Here's how the part is built. I have some questions about the finished solid (model axes, mm). A direction names the side the tool comes from. Coordinates: 2 decimals unless noted, no trailing zeros. Write each loop counter-clockwise with the first axis right and the second up, starting at its lowest first coordinate (ties: lowest second). Pieces come first, ordered by that corner, then holes.
Item 1: I want a section at A-A (x = -2). Please give me the cut outline in (y, z).
Item 2: I want a section at D-D (z = 19). Please give me the cut outline in (x, y).
Item 3: I'm going to push flat-ended pins straight in: P1, Ø5, axis at x = -6, z = -18.5, coming from the +Y side; P2, Ø6, axis at x = -18.5, z = 17, coming from the +Y side; P3, Ø11, axis at y = 12, z = 3, coming from the -X side; P4, Ø10, axis at x = -8.5, y = -3, coming from the -Z side. Where does each tip first touch, or does it pass through?
Item 4: If we mould it in two halves opening along Z, with no side actions, what happens to faces 4 (the face through (22.01, -2.96, -0.33)), 5 (the face through (0, 17, 6.5)), 6 (the face through (-0.28, 9.12, -13.9))? For each: pulls with the +Z half, pulls with the -Z half, needs draft (parallel to the pull), parting line crosses it, or undercut.
Item 5: For faces 1 (the face through (17.46, 7.03, 0.28)), 2 (the face through (-0.3, -2.96, -19.71)), 3 (the face through (11, 13, 0)), which set-ups out of +Z, -Z, +X, -X, +Y, -Y let a thin tool reach every point of the face, with its end or its side?
Item 6: Please list where these lines run through material, in increasing order: line 1 (Z direction, x = 8, y = -0.5); line 2 (Z direction, x = 19, y = -3.25); line 3 (X direction, y = 3, z = 15).
Item 7: I want a section at C-C (y = 5.75). Please give me the cut outline in (x, z), and give its area (3 significant figures).
Item 8: I want a section at B-B (z = -3.5). Please give me the cut outline in (x, y).
from build123d import *
from OCP.BRepFilletAPI import BRepFilletAPI_MakeChamfer

# Parameters (mm, degrees)
SKETCH1_W               = 40
SKETCH1_H               = 40
BOSS_EXTRUDE1_DEPTH     = 8.5
BOSS_EXTRUDE1_TAPER     = 40
SKETCH2_W               = 36
SKETCH2_H               = 36
CUT_EXTRUDE1_DEPTH      = 15
CUT_EXTRUDE1_DRAFT      = -40
SKETCH4_W               = 25.73530627
SKETCH4_H               = 25.73530627
BOSS_EXTRUDE3_DEPTH     = 10
SKETCH5_W               = 22
SKETCH5_H               = 13
CUT_EXTRUDE2_DEPTH      = 31.000000133
CHAMFER2_SIZE           = 12
CHAMFER2_SIZE_2         = 9.89892863
CUT_EXTRUDE3_DEPTH      = 35.154586706
CUT_EXTRUDE3_DEPTH_BACK = 35.154586706
CHAMFER3_SIZE           = 4.3
CHAMFER3_SIZE2          = 7.447818473
CUT_EXTRUDE4_DEPTH      = 35.154586706
CUT_EXTRUDE4_DEPTH_BACK = 35.154586706
SKETCH9_W               = 40.602605658
SKETCH9_H               = 40
BOSS_EXTRUDE4_DEPTH     = 6
BOSS_EXTRUDE4_DRAFT     = -30
SKETCH10_W              = 36.602605658
SKETCH10_H              = 36
CUT_EXTRUDE5_DEPTH      = 10
CUT_EXTRUDE5_DRAFT      = 30


with BuildPart() as part:
    # Sketch1 → Boss-Extrude1 (new body)
    with BuildSketch(Plane(origin=(0, 0, 0), x_dir=(1, 0, 0), z_dir=(0, 1, 0))):
        Rectangle(SKETCH1_W, SKETCH1_H)
    extrude(amount=BOSS_EXTRUDE1_DEPTH, taper=BOSS_EXTRUDE1_TAPER)


with BuildPart() as cut_extrude1_tool:
    # Sketch2 → Cut-Extrude1 (with draft: the straight prism first)
    with BuildSketch(Plane.XZ):
        Rectangle(SKETCH2_W, SKETCH2_H)
    extrude(amount=-CUT_EXTRUDE1_DEPTH)
    # Cut-Extrude1: the draft: its side faces are tilted about the plane it starts from
    cut_extrude1_sides = [cut_extrude1_tool.faces().sort_by_distance(p)[0] for p in [
        (0, 7.5, -18),
        (18, 7.5, 0),
        (0, 7.5, 18),
        (-18, 7.5, 0),
    ]]
    draft(cut_extrude1_sides, Plane.XZ, CUT_EXTRUDE1_DRAFT)


with BuildPart() as part_1:
    add(part.part)

    # Cut-Extrude1: cut by cut_extrude1_tool
    add(cut_extrude1_tool.part, mode=Mode.SUBTRACT)

    # Sketch4 → Boss-Extrude3 (add)
    with BuildSketch(Plane(origin=(0, 8.5, 0), x_dir=(1, 0, 0), z_dir=(0, 1, 0))):
        Rectangle(SKETCH4_W, SKETCH4_H)
    extrude(amount=BOSS_EXTRUDE3_DEPTH)

    # Sketch5 → Cut-Extrude2 (cut, through all)
    with BuildSketch(Plane.XZ.offset(-8.5)):
        Rectangle(SKETCH5_W, SKETCH5_H)
    extrude(amount=-CUT_EXTRUDE2_DEPTH, mode=Mode.SUBTRACT)

    # Chamfer2
    # the kernel refuses this chamfer: 12, 9.89892863 mm, written as the material it adds along each edge
    with BuildSketch(Plane(origin=(12.867653135, 8.5, 44.011128682), x_dir=(0.6427876096865404, -0.7660444431189772, 0), z_dir=(0, 0, -1))) as chamfer2_piece_1_section:
        Polygon((CHAMFER2_SIZE, 0), (-CHAMFER2_SIZE_2 * 0.766044443108, -CHAMFER2_SIZE_2 * 0.642787609677), (0, 0), align=None)
    chamfer2_piece_1 = extrude(amount=88.022257365, mode=Mode.PRIVATE)
    chamfer2_piece_1 = split(chamfer2_piece_1, bisect_by=Plane(origin=(12.867653135, 0, 44.011128682), z_dir=(0, 1, 0)), keep=Keep.TOP, mode=Mode.PRIVATE)
    chamfer2_piece_1 = split(chamfer2_piece_1, bisect_by=Plane(origin=(12.867653135, -0.927920344, 20.676206983), z_dir=(0, -0.37460659341591307, -0.9271838545667871)), keep=Keep.TOP, mode=Mode.PRIVATE)
    chamfer2_piece_1 = split(chamfer2_piece_1, bisect_by=Plane(origin=(12.867653135, 29.644778588, -8.32403482), z_dir=(0, -0.37460659341591274, 0.9271838545667872)), keep=Keep.TOP, mode=Mode.PRIVATE)
    add(chamfer2_piece_1)
    with BuildSketch(Plane(origin=(-12.867653135, 8.5, -44.011128682), x_dir=(-0.6427876096865406, -0.766044443118977, 0), z_dir=(0, 0, 1))) as chamfer2_piece_2_section:
        Polygon((CHAMFER2_SIZE, 0), (-CHAMFER2_SIZE_2 * 0.766044443108, -CHAMFER2_SIZE_2 * 0.642787609677), (0, 0), align=None)
    chamfer2_piece_2 = extrude(amount=88.022257365, mode=Mode.PRIVATE)
    chamfer2_piece_2 = split(chamfer2_piece_2, bisect_by=Plane(origin=(-12.867653135, 0, -44.011128682), z_dir=(0, 1, 0)), keep=Keep.TOP, mode=Mode.PRIVATE)
    chamfer2_piece_2 = split(chamfer2_piece_2, bisect_by=Plane(origin=(-12.867653135, -0.927920344, -20.676206983), z_dir=(0, -0.37460659341591274, 0.9271838545667872)), keep=Keep.TOP, mode=Mode.PRIVATE)
    chamfer2_piece_2 = split(chamfer2_piece_2, bisect_by=Plane(origin=(-12.867653135, 29.644778588, 8.32403482), z_dir=(0, -0.37460659341591307, -0.9271838545667871)), keep=Keep.TOP, mode=Mode.PRIVATE)
    add(chamfer2_piece_2)
    with BuildSketch(Plane(origin=(-44.011128682, 8.5, 12.867653135), x_dir=(0, -0.766044443118977, 0.6427876096865405), z_dir=(1, 0, 0))) as chamfer2_piece_3_section:
        Polygon((CHAMFER2_SIZE, 0), (-CHAMFER2_SIZE_2 * 0.766044443108, -CHAMFER2_SIZE_2 * 0.642787609677), (0, 0), align=None)
    chamfer2_piece_3 = extrude(amount=88.022257365, mode=Mode.PRIVATE)
    chamfer2_piece_3 = split(chamfer2_piece_3, bisect_by=Plane(origin=(-44.011128682, 0, 12.867653135), z_dir=(0, 1, 0)), keep=Keep.TOP, mode=Mode.PRIVATE)
    chamfer2_piece_3 = split(chamfer2_piece_3, bisect_by=Plane(origin=(-20.676206983, -0.927920344, 12.867653135), z_dir=(0.927183854566787, -0.37460659341591307, 0)), keep=Keep.TOP, mode=Mode.PRIVATE)
    chamfer2_piece_3 = split(chamfer2_piece_3, bisect_by=Plane(origin=(8.32403482, 29.644778588, 12.867653135), z_dir=(-0.9271838545667872, -0.37460659341591274, 0)), keep=Keep.TOP, mode=Mode.PRIVATE)
    add(chamfer2_piece_3)
    with BuildSketch(Plane(origin=(44.011128682, 8.5, -12.867653135), x_dir=(0, -0.766044443118977, -0.6427876096865405), z_dir=(-1, 0, 0))) as chamfer2_piece_4_section:
        Polygon((CHAMFER2_SIZE, 0), (-CHAMFER2_SIZE_2 * 0.766044443108, -CHAMFER2_SIZE_2 * 0.642787609677), (0, 0), align=None)
    chamfer2_piece_4 = extrude(amount=88.022257365, mode=Mode.PRIVATE)
    chamfer2_piece_4 = split(chamfer2_piece_4, bisect_by=Plane(origin=(44.011128682, 0, -12.867653135), z_dir=(0, 1, 0)), keep=Keep.TOP, mode=Mode.PRIVATE)
    chamfer2_piece_4 = split(chamfer2_piece_4, bisect_by=Plane(origin=(-8.32403482, 29.644778588, -12.867653135), z_dir=(0.927183854566787, -0.37460659341591307, 0)), keep=Keep.TOP, mode=Mode.PRIVATE)
    chamfer2_piece_4 = split(chamfer2_piece_4, bisect_by=Plane(origin=(20.676206983, -0.927920344, -12.867653135), z_dir=(-0.9271838545667872, -0.37460659341591274, 0)), keep=Keep.TOP, mode=Mode.PRIVATE)
    add(chamfer2_piece_4)

    # Sketch7 → Cut-Extrude3 (cut, two sides: drawn at the far end of the back side and taken through both)
    with BuildSketch(Plane(origin=(0, 0, 0), x_dir=(0, 0, -1), z_dir=(1, 0, 0)).offset(-CUT_EXTRUDE3_DEPTH_BACK)):
        Polygon((-20, 0), (-24.78585356, 0), (-24.78585356, 18.532984169), (-10.14, 18.5), align=None)
    extrude(amount=CUT_EXTRUDE3_DEPTH + CUT_EXTRUDE3_DEPTH_BACK, mode=Mode.SUBTRACT)

    # Chamfer3: one chamfer whose edges measure the first distance from different faces: ONE call of the kernel's chamfer builder (chamfer() names one face for all edges)
    chamfer3_edges_1 = [part_1.edges().sort_by_distance(p)[0] for p in [
        (0, 8.5, 6.5),
    ]]
    chamfer3_side_1 = [part_1.faces().sort_by_distance(p)[0] for p in [
        (0, 8.5, 8.683826567),
    ]]
    chamfer3_edges_2 = [part_1.edges().sort_by_distance(p)[0] for p in [
        (0, 8.5, -6.5),
    ]]
    chamfer3_side_2 = [part_1.faces().sort_by_distance(p)[0] for p in [
        (0, 8.5, -8.683826567),
    ]]
    chamfer3 = BRepFilletAPI_MakeChamfer(part_1.part.solid().wrapped)
    for e in chamfer3_edges_1:
        chamfer3.Add(CHAMFER3_SIZE, CHAMFER3_SIZE2, e.wrapped, chamfer3_side_1[0].wrapped)  # the first distance lies on this face
    for e in chamfer3_edges_2:
        chamfer3.Add(CHAMFER3_SIZE, CHAMFER3_SIZE2, e.wrapped, chamfer3_side_2[0].wrapped)  # the first distance lies on this face
    add(Compound.cast(chamfer3.Shape()), mode=Mode.REPLACE)

    # Sketch8 → Cut-Extrude4 (cut, two sides: drawn at the far end of the back side and taken through both)
    with BuildSketch(Plane(origin=(0, 0, 0), x_dir=(0, 0, -1), z_dir=(1, 0, 0)).offset(-CUT_EXTRUDE4_DEPTH_BACK)):
        Polygon((7.63, 18.5), (12.867653135, 18.5), (21.160182577, 0), (20, 0), align=None)
    extrude(amount=CUT_EXTRUDE4_DEPTH + CUT_EXTRUDE4_DEPTH_BACK, mode=Mode.SUBTRACT)


with BuildPart() as boss_extrude4_tool:
    # Sketch9 → Boss-Extrude4 (with draft: the straight prism first)
    with BuildSketch(Plane.XZ):
        Rectangle(SKETCH9_W, SKETCH9_H)
    extrude(amount=BOSS_EXTRUDE4_DEPTH)
    # Boss-Extrude4: the draft: its side faces are tilted about the plane it starts from
    boss_extrude4_sides = [boss_extrude4_tool.faces().sort_by_distance(p)[0] for p in [
        (0, -3, -20),
        (20.301302829, -3, 0),
        (0, -3, 20),
        (-20.301302829, -3, 0),
    ]]
    draft(boss_extrude4_sides, Plane.XZ, BOSS_EXTRUDE4_DRAFT)


with BuildPart() as part_2:
    add(part_1.part)

    # Boss-Extrude4: add boss_extrude4_tool
    add(boss_extrude4_tool.part)


with BuildPart() as cut_extrude5_tool:
    # Sketch10 → Cut-Extrude5 (with draft: the straight prism first)
    with BuildSketch(Plane(origin=(0, 0, 0), x_dir=(1, 0, 0), z_dir=(0, 1, 0))):
        Rectangle(SKETCH10_W, SKETCH10_H)
    extrude(amount=-CUT_EXTRUDE5_DEPTH)
    # Cut-Extrude5: the draft: its side faces are tilted about the plane it starts from
    cut_extrude5_sides = [cut_extrude5_tool.faces().sort_by_distance(p)[0] for p in [
        (0, -5, 18),
        (18.301302829, -5, 0),
        (0, -5, -18),
        (-18.301302829, -5, 0),
    ]]
    draft(cut_extrude5_sides, Plane(origin=(0, 0, 0), x_dir=(1, 0, 0), z_dir=(0, 1, 0)), CUT_EXTRUDE5_DRAFT)


with BuildPart() as part_3:
    add(part_2.part)

    # Cut-Extrude5: cut by cut_extrude5_tool
    add(cut_extrude5_tool.part, mode=Mode.SUBTRACT)


solid = part_3.part
Answer:
1. outline: (-6, -23.46) - (0, -20) - (18.5, -7.63) - (18.5, -6.5) - (15.95, -6.5) - (8.5, -10.8) - (8.5, -10.87) - (0, -18) - (-6, -21.46) - close; (-6, 21.46) - (0, 18) - (8.5, 10.87) - (8.5, 10.8) - (15.95, 6.5) - (18.5, 6.5) - (18.5, 10.14) - (0, 20) - (-6, 23.46) - close
2. outline: (-23.77, -6) - (-21.77, -6) - (-19.3, -1.73) - (19.3, -1.73) - (21.77, -6) - (23.77, -6) - (20.3, 0) - (19.54, 1.88) - (-19.54, 1.88) - (-20.3, 0) - close
3. P1: stops at y = 5.98
3. P2: stops at y = 9.65
3. P3: stops at x = -17.68
3. P4: stops at z = -23.46
4. face 4: needs draft
4. face 5: undercut
4. face 6: pulls with the -Z half
5. face 1: +Z, -Z, +X, +Y
5. face 2: -Y
5. face 3: +Y
6. line 1: z = -20.29 to -18.29, 18.29 to 20.29
6. line 2: z = -21.88 to -19.88, 19.88 to 21.88
6. line 3: x = -19.09 to -15.48, 15.48 to 19.09
7. outline: (-17.98, -16.16) - (17.98, -16.16) - (17.98, 16.94) - (-17.98, 16.94) - close; hole (-13.18, -13.18) - (13.18, -13.18) - (13.18, 13.18) - (-13.18, 13.18) - close
7. area: 495 mm2
8. outline: (-23.77, -6) - (-21.77, -6) - (-18.3, 0) - (-18, 0) - (-10.87, 8.5) - (-11, 8.5) - (-11, 18.5) - (-12.87, 18.5) - (-12.87, 18.4) - (-20.3, 0) - close; (10.87, 8.5) - (18, 0) - (18.3, 0) - (21.77, -6) - (23.77, -6) - (20.3, 0) - (12.87, 18.4) - (12.87, 18.5) - (11, 18.5) - (11, 8.5) - close
